```python
from build123d import *

# Parameters (mm, degrees)
SKETCH4_W            = 25.1
SKETCH4_H            = 28.75
BOSS_EXTRUDE2_DEPTH  = 53
SKETCH5_W            = 19.1
SKETCH5_H            = 22.75
CUT_EXTRUDE1_DEPTH   = 21.67
FILLET1_R            = 4.1
SKETCH6_W            = 5
SKETCH6_H            = 8
CUT_EXTRUDE2_DEPTH   = 4.67
SKETCH7_W            = 16.769550268
SKETCH7_H            = 35.14
CUT_EXTRUDE3_DEPTH   = 40
SKETCH8_W            = 13.798322684
SKETCH8_H            = 35.14
CUT_EXTRUDE4_DEPTH   = 40
BOSS_EXTRUDE3_DEPTH  = 17
SKETCH10_W           = 3
SKETCH10_H           = 9
BOSS_EXTRUDE4_DEPTH  = 13.8
SKETCH11_W           = 3
SKETCH11_H           = 9
BOSS_EXTRUDE5_DEPTH  = 13.8
SKETCH12_W           = 3
SKETCH12_H           = 12
BOSS_EXTRUDE6_DEPTH  = 16.77
SKETCH24_R           = 1.5
CUT_EXTRUDE6_DEPTH   = 40.8
SKETCH25_W           = 28.75
SKETCH25_H           = 21.925089144
CUT_EXTRUDE7_DEPTH   = 40.8
SKETCH26_W           = 11.913987102
SKETCH26_H           = 12
CUT_EXTRUDE8_DEPTH   = 40.8
SKETCH30_W           = 28.75
SKETCH30_H           = 5.07
BOSS_EXTRUDE10_DEPTH = 30
SKETCH32_W           = 5.990224866
SKETCH32_H           = 23.810252184
BOSS_EXTRUDE13_DEPTH = 30
CUT_EXTRUDE9_DEPTH   = 30
SKETCH36_W           = 5
SKETCH36_H           = 28.75
CUT_EXTRUDE10_DEPTH  = 30
SKETCH38_W           = 5.99
SKETCH38_H           = 5.07
CUT_EXTRUDE11_DEPTH  = 25
SKETCH39_R           = 1.5
CUT_EXTRUDE12_DEPTH  = 25
SKETCH40_R           = 1.5
CUT_EXTRUDE13_DEPTH  = 25
FILLET4_R            = 3
FILLET5_R            = 3
FILLET7_R            = 1


with BuildPart() as part:
    # Sketch4 → Boss-Extrude2 (new body)
    with BuildSketch(Plane(origin=(0, 0, 0), x_dir=(1, 0, 0), z_dir=(0, 1, 0))):
        Rectangle(SKETCH4_W, SKETCH4_H)
    extrude(amount=BOSS_EXTRUDE2_DEPTH)

    # Sketch5 → Cut-Extrude1 (cut)
    with BuildSketch(Plane(origin=(0, 0, 0), x_dir=(-1, 0, 0), z_dir=(0, -1, 0))):
        Rectangle(SKETCH5_W, SKETCH5_H)
    extrude(amount=-CUT_EXTRUDE1_DEPTH, mode=Mode.SUBTRACT)

    # Fillet1
    fillet1_edges = [part.edges().sort_by_distance(p)[0] for p in [
        (0, 21.67, -11.375),
        (0, 21.67, 11.375),
    ]]
    fillet(fillet1_edges, radius=FILLET1_R)

    # Sketch6 → Cut-Extrude2 (cut)
    with BuildSketch(Plane(origin=(0, 21.67, 0), x_dir=(-1, 0, 0), z_dir=(0, -1, 0))):
        Rectangle(SKETCH6_W, SKETCH6_H)
    extrude(amount=-CUT_EXTRUDE2_DEPTH, mode=Mode.SUBTRACT)

    # Sketch7 → Cut-Extrude3 (cut)
    with BuildSketch(Plane(origin=(12.55, 0, 0), x_dir=(0, 0, -1), z_dir=(1, 0, 0))):
        Rectangle(SKETCH7_W, SKETCH7_H)
    extrude(amount=-CUT_EXTRUDE3_DEPTH, mode=Mode.SUBTRACT)

    # Sketch8 → Cut-Extrude4 (cut)
    with BuildSketch(Plane(origin=(0, 0, -14.375), x_dir=(-1, 0, 0), z_dir=(0, 0, -1))):
        Rectangle(SKETCH8_W, SKETCH8_H)
    extrude(amount=-CUT_EXTRUDE4_DEPTH, mode=Mode.SUBTRACT)

    # Sketch9 → Boss-Extrude3 (add)
    with BuildSketch(Plane.XZ):
        Polygon((-9.55, 8.384775134), (-12.55, 8.384775134), (-12.55, 14.375), (-6.899161342, 14.375), (-6.899161342, 11.375), (-9.55, 11.375), align=None)
        Polygon((-9.55, -8.384775134), (-12.55, -8.384775134), (-12.55, -14.375), (-6.899161342, -14.375), (-6.899161342, -11.375), (-9.55, -11.375), align=None)
        Polygon((6.899161342, -11.375), (6.899161342, -14.375), (12.55, -14.375), (12.55, -8.384775134), (9.55, -8.384775134), (9.55, -11.375), align=None)
        Polygon((9.55, 8.384775134), (12.55, 8.384775134), (12.55, 14.375), (6.899161342, 14.375), (6.899161342, 11.375), (9.55, 11.375), align=None)
    extrude(amount=BOSS_EXTRUDE3_DEPTH)

    # Sketch10 → Boss-Extrude4 (add)
    with BuildSketch(Plane(origin=(-6.899161342, 0, 0), x_dir=(0, 0, -1), z_dir=(1, 0, 0))):
        with Locations((-12.875, -12.5)):
            Rectangle(SKETCH10_W, SKETCH10_H)
    extrude(amount=BOSS_EXTRUDE4_DEPTH)

    # Sketch11 → Boss-Extrude5 (add)
    with BuildSketch(Plane.ZY.offset(-6.899161342)):
        with Locations((-12.875, -12.5)):
            Rectangle(SKETCH11_W, SKETCH11_H)
    extrude(amount=BOSS_EXTRUDE5_DEPTH)

    # Sketch12 → Boss-Extrude6 (add)
    with BuildSketch(Plane.XY.offset(-8.384775134)):
        with Locations((-11.05, -11)):
            Rectangle(SKETCH12_W, SKETCH12_H)
        with Locations((11.05, -11)):
            Rectangle(SKETCH12_W, SKETCH12_H)
    extrude(amount=BOSS_EXTRUDE6_DEPTH)

    # Sketch24 → Cut-Extrude6 (cut)
    with BuildSketch(Plane(origin=(12.55, 0, 0), x_dir=(0, 0, -1), z_dir=(1, 0, 0))):
        with Locations((8.675, -11.18)):
            Circle(SKETCH24_R)
        with Locations((-9.075, -11.18)):
            Circle(SKETCH24_R)
    extrude(amount=-CUT_EXTRUDE6_DEPTH, mode=Mode.SUBTRACT)

    # Sketch25 → Cut-Extrude7 (cut)
    with BuildSketch(Plane.ZY.offset(12.55)):
        with Locations((0, 42.037455428)):
            Rectangle(SKETCH25_W, SKETCH25_H)
    extrude(amount=-CUT_EXTRUDE7_DEPTH, mode=Mode.SUBTRACT)

    # Sketch26 → Cut-Extrude8 (cut)
    with BuildSketch(Plane.ZY.offset(12.55)):
        with Locations((0.21531302, -11)):
            Rectangle(SKETCH26_W, SKETCH26_H)
    extrude(amount=-CUT_EXTRUDE8_DEPTH, mode=Mode.SUBTRACT)

    # Sketch30 → Boss-Extrude10 (add)
    with BuildSketch(Plane(origin=(12.55, 0, 0), x_dir=(0, 0, -1), z_dir=(1, 0, 0))):
        with Locations((0, 28.539910856)):
            Rectangle(SKETCH30_W, SKETCH30_H)
    extrude(amount=BOSS_EXTRUDE10_DEPTH)

    # Sketch32 → Boss-Extrude13 (add)
    with BuildSketch(Plane(origin=(12.55, 0, 0), x_dir=(0, 0, -1), z_dir=(1, 0, 0))):
        with Locations((-11.379887567, 3.799784764)):
            Rectangle(SKETCH32_W, SKETCH32_H)
        with Locations((11.379887567, 3.799784764)):
            Rectangle(SKETCH32_W, SKETCH32_H)
    extrude(amount=BOSS_EXTRUDE13_DEPTH)

    # Sketch35 → Cut-Extrude9 (cut)
    with BuildSketch(Plane(origin=(0, 0, -14.375), x_dir=(-1, 0, 0), z_dir=(0, 0, -1))):
        Polygon((-42.55, 11.704910856), (-27.55, 11.704910856), (-12.55, -8.105341328), (-42.55, -8.105341328), align=None)
    extrude(amount=-CUT_EXTRUDE9_DEPTH, mode=Mode.SUBTRACT)

    # Sketch36 → Cut-Extrude10 (cut)
    with BuildSketch(Plane(origin=(0, 31.074910856, 0), x_dir=(1, 0, 0), z_dir=(0, 1, 0))):
        with Locations((40.05, 0)):
            Rectangle(SKETCH36_W, SKETCH36_H)
    extrude(amount=-CUT_EXTRUDE10_DEPTH, mode=Mode.SUBTRACT)

    # Sketch38 → Cut-Extrude11 (cut)
    with BuildSketch(Plane(origin=(37.55, 0, 0), x_dir=(0, 0, -1), z_dir=(1, 0, 0))):
        with Locations((-11.38, 28.539910856)):
            Rectangle(SKETCH38_W, SKETCH38_H)
        with Locations((11.38, 28.539910856)):
            Rectangle(SKETCH38_W, SKETCH38_H)
    extrude(amount=-CUT_EXTRUDE11_DEPTH, mode=Mode.SUBTRACT)

    # Sketch39 → Cut-Extrude12 (cut)
    with BuildSketch(Plane(origin=(0, 11.704910856, 0), x_dir=(-1, 0, 0), z_dir=(0, -1, 0))):
        with Locations(Location((-33.55, 11.379887567, 0), (0, 0, 90))):
            Circle(SKETCH39_R)
        with Locations(Location((-33.55, -11.379887567, 0), (0, 0, 90))):
            Circle(SKETCH39_R)
    extrude(amount=-CUT_EXTRUDE12_DEPTH, mode=Mode.SUBTRACT)

    # Sketch40 → Cut-Extrude13 (cut)
    with BuildSketch(Plane.XZ.offset(-26.004910856)):
        with Locations(Location((31.55, 0, 0), (0, 0, 270))):
            Circle(SKETCH40_R)
    extrude(amount=-CUT_EXTRUDE13_DEPTH, mode=Mode.SUBTRACT)

    # Fillet4
    fillet4_edges = [part.edges().sort_by_distance(p)[0] for p in [
        (-12.55, 31.074910856, 0),
        (0, 31.074910856, 14.375),
        (0, 31.074910856, -14.375),
    ]]
    fillet(fillet4_edges, radius=FILLET4_R)

    # Fillet5
    # the kernel refuses this fillet: 3 mm, written as the material it takes off along each edge
    with BuildSketch(Plane(origin=(-9.55, 28.074910856, 11.375), x_dir=(0, 0, 1), z_dir=(-1, 0, 0))) as fillet5_piece_1_section:
        Polygon((0, 0), (FILLET5_R, 0), (FILLET5_R, FILLET5_R), (0, FILLET5_R), align=None)
    fillet5_piece_1 = extrude(amount=FILLET5_R, mode=Mode.PRIVATE)
    fillet5_piece_1 = fillet5_piece_1 - Plane(origin=(-9.55, 28.074910856, 11.375), x_dir=(0, -0.7071067811865475, -0.7071067811865475), z_dir=(-1, 0, 0)) * Sphere(FILLET5_R, mode=Mode.PRIVATE)
    add(fillet5_piece_1, mode=Mode.SUBTRACT)
    with BuildSketch(Plane(origin=(-9.55, 28.074910856, -11.375), x_dir=(-1, 0, 0), z_dir=(0, 0, -1))) as fillet5_piece_2_section:
        Polygon((0, 0), (FILLET5_R, 0), (FILLET5_R, FILLET5_R), (0, FILLET5_R), align=None)
    fillet5_piece_2 = extrude(amount=FILLET5_R, mode=Mode.PRIVATE)
    fillet5_piece_2 = fillet5_piece_2 - Plane(origin=(-9.55, 28.074910856, -11.375), x_dir=(0.7071067811865475, -0.7071067811865475, 0), z_dir=(0, 0, -1)) * Sphere(FILLET5_R, mode=Mode.PRIVATE)
    add(fillet5_piece_2, mode=Mode.SUBTRACT)
    with BuildSketch(Plane(origin=(-12.55, 28.074910856, -14.375), x_dir=(1, 0, 0), z_dir=(0, -1, 0))) as fillet5_piece_3:
        with BuildLine():
            CenterArc((FILLET5_R, FILLET5_R), FILLET5_R, 180, 90)
            Line((0, FILLET5_R), (0, 0))
            Line((0, 0), (FILLET5_R, 0))
        make_face()
    extrude(amount=52.574910856, mode=Mode.SUBTRACT)
    with BuildSketch(Plane(origin=(-12.55, -24.5, 14.375), x_dir=(0, 0, -1), z_dir=(0, 1, 0))) as fillet5_piece_4:
        with BuildLine():
            CenterArc((FILLET5_R, -FILLET5_R), FILLET5_R, 90, 90)
            Line((0, -FILLET5_R), (0, 0))
            Line((0, 0), (FILLET5_R, 0))
        make_face()
    extrude(amount=52.574910856, mode=Mode.SUBTRACT)

    # Fillet7
    fillet7_edges = [part.edges().sort_by_distance(p)[0] for p in [
        (37.55, 13.704910856, -14.375),
        (37.55, 13.704910856, -8.384775134),
        (37.55, 13.704910856, 14.375),
        (37.55, 13.704910856, 8.384775134),
    ]]
    fillet(fillet7_edges, radius=FILLET7_R)


solid = part.part
```
Geometry: final body of the model. Coordinates: model frame, mm. A direction names the side the tool comes from. Round coordinates to 2 decimals unless told otherwise and drop trailing zeros. Order: outer loops, then holes, each group sorted by start corner. A loop starts at its lowest first (then second) coordinate and runs counter-clockwise, first axis right, second up. Notation, with made-up numbers: M 3,45.5 L 18,45.5 A23 cw 18,82.5 Z; hole C -24.5,31 d7. An arc over 180 degrees is marked long. One line per item, written item: value.
(1) Pin query (flat end, axial travel): P1, Ø3, axis at y = 17.5, z = -1, coming from the +X side; P2, Ø6.5, axis at x = 31.5, z = -11, coming from the -Y side; P3, Ø5, axis at x = 30, z = 10.5, coming from the -Y side. Return the tip coordinate at first contact, or that it passes through.
Result sheet:
P1: x = 12.55
P2: y = 11.7
P3: y = 11.64
(2) Cut plane B-B (x = -5). Return the cut outline in (y, z) (3 decimals).
Result sheet:
outline: M -17,-14.375 L -8,-14.375 L -8,-11.375 L -17,-11.375 Z; M -17,11.375 L -8,11.375 L -8,14.375 L -17,14.375 Z; M 17.57,-14.375 L 28.075,-14.375 A3 ccw 31.075,-11.375 L 31.075,11.375 A3 ccw 28.075,14.375 L 17.57,14.375 L 17.57,11.375 A4.1 cw 21.67,7.275 L 21.67,-7.275 A4.1 cw 17.57,-11.375 Z
(3) Reachability of faces 5 (the flat face through (0, 17.57, -13)), 6 (the cylindrical face through (-11.695, 30.173, 0.159)), 7 (the flat face through (11, 17.57, 0)), 8 (the flat face through (11, -11, 6.172)), 9 (the flat face through (31.5, 11.705, -11.4)) from +Z, -Z, +X, -X, +Y, -Y: full face, straight path, thin tool, end or side. Return the list, or none.
Result sheet:
face 5: +Z, -Z
face 6: +Z, -Z, -X, +Y
face 7: +X, -X
face 8: +X, -X, -Y
face 9: +Z, -Z, +X, -Y
(4) Line query: probe 1 along Z at (x, y) = (11, -11) (3 decimals); probe 2 along Z at (x, y) = (7, -12) (3 decimals); probe 3 along X at (y, z) = (-0.5, 11.5). Output: solid intervals per line, ascending. Write a range as [from, to].
Result sheet:
probe 1: [-14.375, -10.164], [-7.186, -5.742], [6.172, 7.586], [10.564, 14.375]
probe 2: [-14.375, -11.375], [11.375, 14.375]
probe 3: [-12.55, -6.9], [6.9, 18.31]
(5) Pull-direction query (Z, two-part tool) for faces 1 (the flat face through (0, -8, 13)), 2 (the flat face through (8, 5, 14.375)), 3 (the flat face through (9.55, 7, 9)), 4 (the cylindrical face through (11.07, -12.51, 8.38)); classes: pulls with the +Z half, pulls with the -Z half, needs draft (parallel to the pull), parting line crosses it, or undercut.
Result sheet:
face 1: needs draft
face 2: pulls with the +Z half
face 3: undercut
face 4: undercut
(6) Cut plane A-A (y = -11.18). Give the number of separate pieces and of enclosed holes in the cut face, and give its area (3 significant figures).
Result sheet:
separate pieces: 6
enclosed holes: 0
area: 176 mm2
(7) Cut plane D-D (y = 25). Return the cut outline in (x, z) (3 decimals).
Result sheet:
outline: M -12.55,-11.375 A3 ccw -9.55,-14.375 L 12.55,-14.375 L 12.55,14.375 L -9.55,14.375 A3 ccw -12.55,11.375 Z; hole M -2.5,-4 L 2.5,-4 L 2.5,4 L -2.5,4 Z
(8) Cut plane C-C (z = 0). Return the cut outline in (x, y).
Result sheet:
outline: M -12.55,17.57 L -9.55,17.57 L -9.55,21.67 L -2.5,21.67 L -2.5,26.34 L 2.5,26.34 L 2.5,21.67 L 9.55,21.67 L 9.55,17.57 L 12.55,17.57 L 12.55,26 L 30.05,26 L 30.05,31.07 L -9.55,31.07 A3 ccw -12.55,28.07 Z; M 33.05,26 L 37.55,26 L 37.55,31.07 L 33.05,31.07 Z
